Geometry check sheet. Reference: the model listing, model coordinates, mm. Face numbers are marked on the shaded views. A direction names the side the tool comes from. Coordinates: 2 decimals unless noted, no trailing zeros. Loops run counter-clockwise (first coordinate to the right, second up) from the corner with the lowest first, then second, coordinate; pieces in that order, holes last. Notation, with made-up numbers: M 34.25,59.5 L 78.25,59.5 A35 ccw 78.25,94.5 Z; hole C 2.5,20.5 d3. An arc over 180 degrees is marked long. Use CSV: the item, a comma, the result in double quotes.
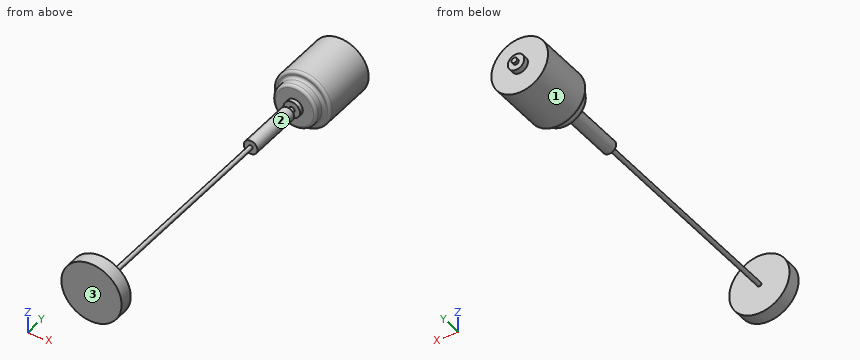
```python
from build123d import *

# Parameters (mm, degrees)
CROQUIS2_R              = 3
SALIENTE_EXTRUIR1_DEPTH = 2
CROQUIS3_R              = 1
SALIENTE_EXTRUIR2_DEPTH = 1
SALIENTE_EXTRUIR3_START = 2.5
CROQUIS4_R              = 1
SALIENTE_EXTRUIR3_DEPTH = 2.5
CROQUIS5_R              = 2.5
SALIENTE_EXTRUIR4_DEPTH = 20
CROQUIS6_R              = 0.75
SALIENTE_EXTRUIR5_DEPTH = 82
CROQUIS7_R              = 11
SALIENTE_EXTRUIR6_DEPTH = 5
REDONDEO1_R             = 1


with BuildPart() as part:
    # Croquis1 → Revolución1 (revolve)
    with BuildSketch(Plane.XY, mode=Mode.PRIVATE) as revoluci_n1_sk:
        Polygon((0, 0), (0, 26.5), (10.35, 26.5), (10.35, 5.5), (7.9, 5.5), (7.9, 1.5), (3, 1.5), (3, 0), align=None)
    revolve(revoluci_n1_sk.sketch.rotate(Axis((0, 14.951468567, 0), (0, 1, 0)), 90), axis=Axis((0, 14.951468567, 0), (0, 1, 0)))

    # Croquis2 → Saliente-Extruir1 (add)
    with BuildSketch(Plane(origin=(0, 26.5, 0), x_dir=(1, 0, 0), z_dir=(0, 1, 0))):
        with Locations(Location((0, 0, 0), (0, 0, 90))):
            Circle(CROQUIS2_R)
    extrude(amount=SALIENTE_EXTRUIR1_DEPTH)

    # Croquis3 → Saliente-Extruir2 (add)
    with BuildSketch(Plane(origin=(0, 28.5, 0), x_dir=(1, 0, 0), z_dir=(0, 1, 0))):
        with Locations(Location((0, 0, 0), (0, 0, 270))):
            Circle(CROQUIS3_R)
    extrude(amount=SALIENTE_EXTRUIR2_DEPTH)

    # Croquis4 → Saliente-Extruir3 (add)
    with BuildSketch(Plane.XZ.offset(SALIENTE_EXTRUIR3_START)):
        with Locations(Location((0, 0, 0), (0, 0, 90))):
            Circle(CROQUIS4_R)
    extrude(amount=-SALIENTE_EXTRUIR3_DEPTH)

    # Croquis5 → Saliente-Extruir4 (add)
    with BuildSketch(Plane.XZ.offset(2.5)):
        with Locations(Location((0, 0, 0), (0, 0, 270))):
            Circle(CROQUIS5_R)
    extrude(amount=SALIENTE_EXTRUIR4_DEPTH)

    # Croquis6 → Saliente-Extruir5 (add)
    with BuildSketch(Plane.XZ.offset(22.5)):
        with Locations(Location((0, 0, 0), (0, 0, 270))):
            Circle(CROQUIS6_R)
    extrude(amount=SALIENTE_EXTRUIR5_DEPTH)

    # Croquis7 → Saliente-Extruir6 (add)
    with BuildSketch(Plane.XZ.offset(104.5)):
        with Locations(Location((0, 0, 0), (0, 0, 270))):
            Circle(CROQUIS7_R)
    extrude(amount=SALIENTE_EXTRUIR6_DEPTH)

    # Redondeo1
    redondeo1_edges = [part.edges().sort_by_distance(p)[0] for p in [
        (0, 1.5, 7.9),
        (0, 5.5, 7.9),
        (0, 5.5, 10.35),
    ]]
    fillet(redondeo1_edges, radius=REDONDEO1_R)


solid = part.part
```
1. Section check A-A, the plane y = -16. Record the cut outline in (x, z), plus the area to 3 significant figures.
The answers:
outline,"C 0,0 d5"
area,"19.6 mm^2"
2. Thickness scan on line 1 (Y direction, x = -5.5, z = 3.75); line 2 (X direction, y = -58, z = 0); line 3 (Y direction, x = 4.25, z = -6.75). Record the ranges inside material, lowest first. Write a range as [from, to].
The answers:
line 1,"[-109.5, -104.5], [1.5, 26.5]"
line 2,"[-0.75, 0.75]"
line 3,"[-109.5, -104.5], [4.88, 26.5]"
3. Gauge pin test, flat ends, axial feed: P1, Ø12, axis at y = -57, z = -2.5, coming from the -X side; P2, Ø5, axis at x = 4, z = -6.5, coming from the +Y side; P3, Ø6, axis at x = -5, z = 0.5, coming from the +Y side; P4, Ø10, axis at y = -76.5, z = -6, coming from the -X side. Record the tip position at first contact, or that the pin passes through.
The answers:
P1,"x = -0.75"
P2,"y = 26.5"
P3,"y = 28.5"
P4,"through"
4. Section check B-B, the plane y = -62. Record the cut outline in (x, z), plus the area to 3 significant figures.
The answers:
outline,"C 0,0 d1.5"
area,"1.77 mm^2"
5. Set-up check for the marked faces 1, 2 and 3: record each of +Z, -Z, +X, -X, +Y, -Y from which the full face is reachable in a straight line by a thin tool's end or side.
The answers:
face 1,"+Y"
face 2,"none"
face 3,"+Z, -Z, +X, -X, -Y"
